Can you work these out from the model? Positions are in its coordinate system, mm. A direction names the side the tool comes from. Give positions to 0.01 mm unless a question says otherwise; leave off trailing zeros. Loops run counter-clockwise (first coordinate to the right, second up) from the corner with the lowest first, then second, coordinate; pieces in that order, holes last. Notation, with made-up numbers: (46, -14) - (53, -14) arc R13 ccw to (53, -3) - close; hole circle Ø5 at (-3, -7). An arc over 180 degrees is marked (long way). Answer as a JSON object with one key per item and string values.
```python
from build123d import *

# Parameters (mm, degrees)
SKETCH1_W                      = 114.3
SKETCH1_H                      = 114.3
BOSS_EXTRUDE1_DEPTH            = 10.16
CBORE_FOR_M6_SHCS1_D           = 6.6
CBORE_FOR_M6_SHCS1_CBORE_D     = 9.4
CBORE_FOR_M6_SHCS1_CBORE_DEPTH = 6.4
SKETCH6_R                      = 4.2164
CUT_EXTRUDE1_DEPTH             = 13.97


with BuildPart() as part:
    # Sketch1 → Boss-Extrude1 (new body)
    with BuildSketch(Plane(origin=(0, 0, 0), x_dir=(1, 0, 0), z_dir=(0, 1, 0))):
        Rectangle(SKETCH1_W, SKETCH1_H)
    extrude(amount=BOSS_EXTRUDE1_DEPTH)

    # CBORE for M6 SHCS1 (through all)
    with Locations(Plane(origin=(0, 10.16, 0), x_dir=(1, 0, 0), z_dir=(0, 1, 0))):
        with Locations((-25.4, 25.4), (25.4, 25.4), (25.4, -25.4), (-25.4, -25.4)):
            CounterBoreHole(CBORE_FOR_M6_SHCS1_D / 2, CBORE_FOR_M6_SHCS1_CBORE_D / 2, CBORE_FOR_M6_SHCS1_CBORE_DEPTH)

    # Sketch6 → Cut-Extrude1 (cut)
    with BuildSketch(Plane(origin=(57.15, 0, 0), x_dir=(0, 0, -1), z_dir=(1, 0, 0))):
        with Locations((0, 5.08)):
            Circle(SKETCH6_R)
    extrude(amount=-CUT_EXTRUDE1_DEPTH, mode=Mode.SUBTRACT)


solid = part.part
```
1) I'm going to push flat-ended pins straight in: P1, Ø7.5, axis at x = -25, z = -23, coming from the +Y side; P2, Ø8.5, axis at x = -25.4, z = -25.4, coming from the +Y side; P3, Ø2.5, axis at y = 4.5, z = 0, coming from the +X side; P4, Ø5.5, axis at x = 25.4, z = 25.4, coming from the +Y side. Where does each tip first touch, or does it pass through?
Check sheet entries:
{"P1": "y = 10.16", "P2": "y = 3.76", "P3": "x = 43.18", "P4": "through"}
2) Imagine slicing it at B-B on x = -25.4. Write out the boundary of the cut face in (y, z), and give its area (3 significant figures).
Check sheet entries:
{"outline": "(0, -57.15) - (10.16, -57.15) - (10.16, -30.1) - (3.76, -30.1) - (3.76, -28.7) - (0, -28.7) - close; (0, -22.1) - (3.76, -22.1) - (3.76, -20.7) - (10.16, -20.7) - (10.16, 20.7) - (3.76, 20.7) - (3.76, 22.1) - (0, 22.1) - close; (0, 28.7) - (3.76, 28.7) - (3.76, 30.1) - (10.16, 30.1) - (10.16, 57.15) - (0, 57.15) - close", "area": "991 mm2"}
3) If we mould it in two halves opening along Z, with no side actions, what happens to faces 1 (the flat face through (22, 3.76, -24)), 2 (the flat face through (-57.15, 5, 1)), 3 (the flat face through (-1, 5, -57.15))? For each: released by +Z, released by -Z, zero draft, split by the parting line, or undercut.
Check sheet entries:
{"face 1": "undercut", "face 2": "zero draft", "face 3": "released by -Z"}
4) Imagine slicing it at A-A on z = -25.4. Write out the boundary of the cut face in (x, y), and give its area (3 significant figures).
Check sheet entries:
{"outline": "(-57.15, 0) - (-28.7, 0) - (-28.7, 3.76) - (-30.1, 3.76) - (-30.1, 10.16) - (-57.15, 10.16) - close; (-22.1, 0) - (22.1, 0) - (22.1, 3.76) - (20.7, 3.76) - (20.7, 10.16) - (-20.7, 10.16) - (-20.7, 3.76) - (-22.1, 3.76) - close; (28.7, 0) - (57.15, 0) - (57.15, 10.16) - (30.1, 10.16) - (30.1, 3.76) - (28.7, 3.76) - close", "area": "991 mm2"}
5) Which directions (+Z, -Z, +X, -X, +Y, -Y) give clear straight access to the entire face, cutting with the end or side of a thin tool? Please do faces 4 (the flat face through (-29, 3.76, 26)), 5 (the flat face through (-1, 10.16, -1)), 6 (the cylindrical face through (50.263, 0.964, 0.914)).
Check sheet entries:
{"face 4": "+Y", "face 5": "+Z, -Z, +X, -X, +Y", "face 6": "+X"}
6) Imagine slicing it at D-D on z = 0. Write out the boundary of the cut face in (x, y).
Check sheet entries:
{"outline": "(-57.15, 0) - (57.15, 0) - (57.15, 0.86) - (43.18, 0.86) - (43.18, 9.3) - (57.15, 9.3) - (57.15, 10.16) - (-57.15, 10.16) - close"}
7) I need wall thicknesses on L1, parallel to Z at x = -25.4, y = 1.8; L2, parallel to Z at x = 25.4, y = 7.5. Which ranges of each line are inside material? Lowest first, please.
Check sheet entries:
{"L1": "-57.15 to -28.7, -22.1 to 22.1, 28.7 to 57.15", "L2": "-57.15 to -30.1, -20.7 to 20.7, 30.1 to 57.15"}
8) Imagine slicing it at C-C on x = 47. Write out the boundary of the cut face in (y, z), and give its area (3 significant figures).
Check sheet entries:
{"outline": "(0, -57.15) - (10.16, -57.15) - (10.16, 57.15) - (0, 57.15) - close; hole circle Ø8.43 at (5.08, 0)", "area": "1,110 mm2"}
